from build123d import *

# Parameters (mm, degrees)
EXTRUDE_1_DEPTH = 4


with BuildPart() as part:
    # Sketch 1 → Бобышка-Вытянуть1 (new body)
    with BuildSketch(Plane(origin=(1e-09, -39.529244173, -14.757642275), x_dir=(9.977709055986143e-13, 0.6139406135149353, 0.7893522173763147), z_dir=(1.0, -1.5354534328683506e-11, 1.0678377959596007e-11))):
        Polygon((0, 0), (28.416679826, 22.101862087), (45.607017004, 0), (17.190337178, -22.101862087), align=None)
        Polygon((34.205262753, 11.401754251), (42.800431342, 0.350823208), (31.749500299, -8.244345381), (23.15433171, 2.806585662), align=None, mode=Mode.SUBTRACT)
        Polygon((8.945991797, -8.244345381), (19.99692284, 0.350823208), (28.592091429, -10.700107836), (17.541160386, -19.295276425), align=None, mode=Mode.SUBTRACT)
    extrude(amount=EXTRUDE_1_DEPTH)


solid = part.part
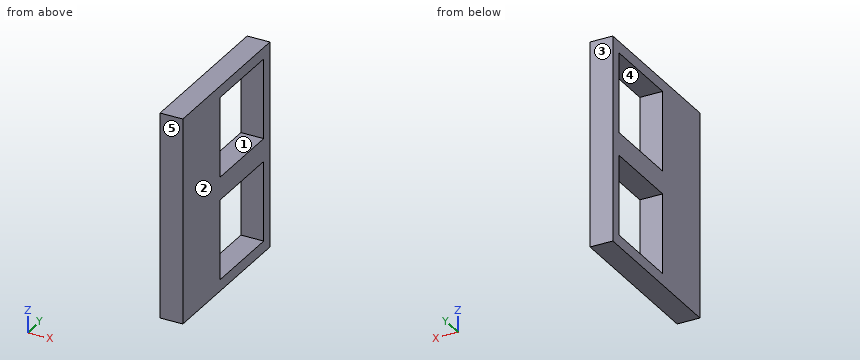
Source: CAD feature listing. Evaluate the final solid. Frame: model axes, mm. Face numbers are marked on the shaded views. A direction names the side the tool comes from. Give positions to 0.01 mm unless a question says otherwise; leave off trailing zeros. Write each loop counter-clockwise with the first axis right and the second up, starting at its lowest first coordinate (ties: lowest second). Pieces come first, ordered by that corner, then holes. Notation, with made-up numbers: M 65.25,-23.5 L 122.25,-23.5 A28 cw 122.25,6.5 Z; hole C -6,59 d5. An arc over 180 degrees is marked long. Return JSON: item names as keys, results as strings. Group by question number.
1) Pin query (flat end, axial travel): P1, Ø1, axis at y = -16.5, z = 5.5, coming from the -X side. Return the tip coordinate at first contact, or that it passes through.
2) Material intervals for line 1 along Z through (x, y) = (2.7, -18.5); line 2 along Y through (x, z) = (1.15, -7), sorted ascending. Write a range as [from, to].
3) Set-up query: the marked faces 1 and 2. Return all of +Z, -Z, +X, -X, +Y, -Y with unobstructed straight access to the full face (end or side cutting, diameter ignored); none if empty.
4) Cut plane A-A, the plane x = 1.65. Output: boundary loops of the cut face in (y, z), plus the area to 3 significant figures.
5) Cut plane B-B, the plane z = 10.5. Output: boundary loops of the cut face in (x, y), plus the area to 3 significant figures.
6) Pull-direction query (Y, two-part tool) for the marked faces 3, 4 and 5; classes: pulls with the +Y half, pulls with the -Y half, needs draft (parallel to the pull), parting line crosses it, or undercut.
7) Cut plane C-C, the plane y = -15.25. Output: boundary loops of the cut face in (x, z), plus the area to 3 significant figures.
Recorded:
{
 "1": {"P1": "stops at x = 0"},
 "2": {"line 1": "z = [-14.76, -12.76], [1.24, 5.24], [19.24, 21.24]", "line 2": "y = [-39.53, -27.53], [-13.53, -11.53]"},
 "3": {"face 1": "+X, -X", "face 2": "+Z, -Z, +X, +Y, -Y"},
 "4": {"outline": "M -39.53,-14.76 L -11.53,-14.76 L -11.53,21.24 L -39.53,21.24 Z; hole M -27.53,-12.76 L -13.53,-12.76 L -13.53,1.24 L -27.53,1.24 Z; hole M -27.53,5.24 L -13.53,5.24 L -13.53,19.24 L -27.53,19.24 Z", "area": "616 mm²"},
 "5": {"outline": "M 0,-39.53 L 4,-39.53 L 4,-27.53 L 0,-27.53 Z; M 0,-13.53 L 4,-13.53 L 4,-11.53 L 0,-11.53 Z", "area": "56.0 mm²"},
 "6": {"face 3": "pulls with the +Y half", "face 4": "undercut", "face 5": "pulls with the -Y half"},
 "7": {"outline": "M 0,-14.76 L 4,-14.76 L 4,-12.76 L 0,-12.76 Z; M 0,1.24 L 4,1.24 L 4,5.24 L 0,5.24 Z; M 0,19.24 L 4,19.24 L 4,21.24 L 0,21.24 Z", "area": "32.0 mm²"}
}
